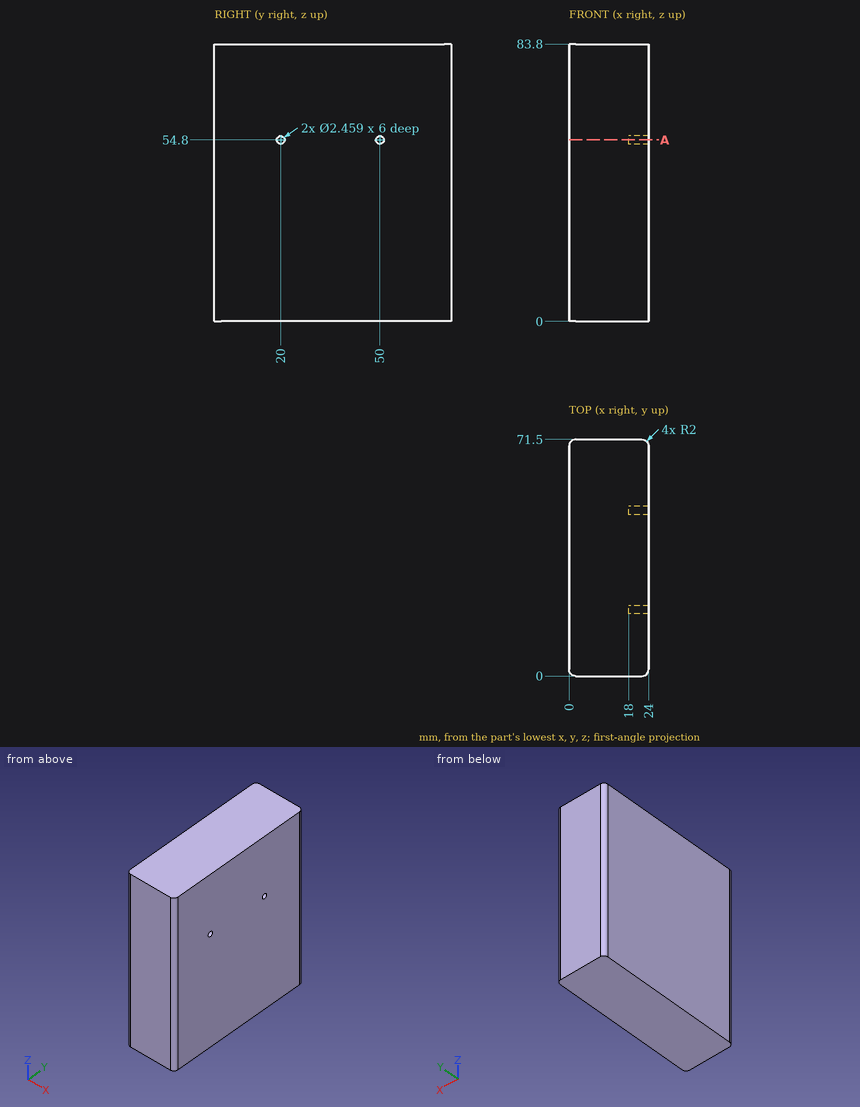
Answer from the drawing. Dimensions are ordinates in mm from the lowest x, y and z of the part. Coordinates: 2 decimals unless noted, no trailing zeros. Order: outer loops, then holes, each group sorted by start corner. A loop starts at its lowest first (then second) coordinate and runs counter-clockwise, first axis right, second up. Notation, with made-up numbers: (6.25, 34.5) - (21.25, 34.5) arc R29 cw to (21.25, 72.5) - close; hole circle Ø10 at (72, 72). An arc over 180 degrees is marked (long way). Answer as a JSON object with one key per item and string values. Group by question number.
Item 1: Flat-ended cylindrical pins translate along their axes: P1, Ø4, axis at x = 11, z = 49.5, coming from the -Y side; P2, Ø0.7, axis at y = 20.5, z = 54.5, coming from the +X side. Find the tip coordinate at first contact, or state that the pin passes through.
Item 2: Consider probe 1 along Y at (x, z) = (19.6, 54.8); probe 2 along Z at (x, y) = (22.2, 20); probe 3 along Y at (x, z) = (22.8, 54.8). Determine where each line is inside the solid, lowest interval first. Write a range as from..to.
Item 3: Section A-A (z = 54.8) is taken. Give the vertices of the cut face in (x, y).
Results are:
{
 "1": {"P1": "stops at y = 0", "P2": "stops at x = 18"},
 "2": {"probe 1": "y = 0..18.77, 21.23..48.77, 51.23..71.5", "probe 2": "z = 0..53.57, 56.03..83.8", "probe 3": "y = 0.17..18.77, 21.23..48.77, 51.23..71.33"},
 "3": {"outline": "(0, 2) arc R2 ccw to (2, 0) - (22, 0) arc R2 ccw to (24, 2) - (24, 18.77) - (18, 18.77) - (18, 21.23) - (24, 21.23) - (24, 48.77) - (18, 48.77) - (18, 51.23) - (24, 51.23) - (24, 69.5) arc R2 ccw to (22, 71.5) - (2, 71.5) arc R2 ccw to (0, 69.5) - close"}
}
